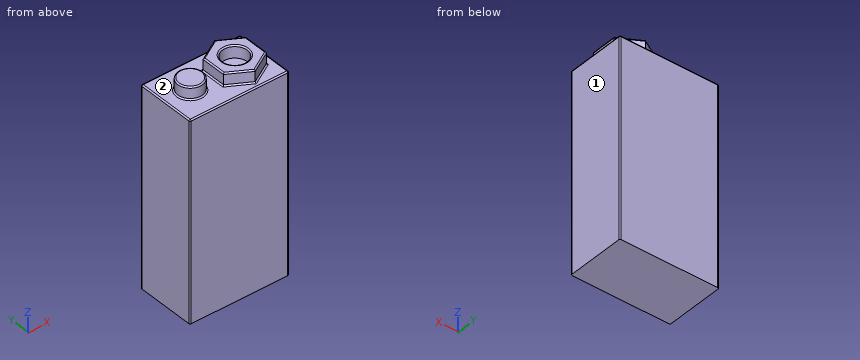
Autodesk Inventor part; units mm, degrees
ref_plane "YZ Plane" through (0, 0, 0) normal (1, 0, 0) x (0, 1, 0)
ref_plane "XZ Plane" through (0, 0, 0) normal (0, 1, 0) x (-1, 0, 0)
ref_plane "XY Plane" through (0, 0, 0) normal (0, 0, 1) x (1, 0, 0)
sketch "Sketch1" plane through (0, 0, 0) normal (0, 0, 1) x (1, 0, 0)
  line L0 (20, 12) -> (0, 12)
  line L1 (0, 12) -> (0, 0)
  line L2 (0, 0) -> (20, 0)
  line L3 (20, 0) -> (20, 12)
extrude "Extrusion1" add sketch "Sketch1" along normal blind 40
sketch "Sketch2" plane through (0, 0, 40) normal (0, 0, 1) x (1, 0, 0)
  circle A0 centre (5, 6) radius 2.5
  line L0 (14, 1) -> (9.6699, 3.5)
  line L1 (9.6699, 3.5) -> (9.6699, 8.5)
  line L2 (9.6699, 8.5) -> (14, 11)
  line L3 (14, 11) -> (18.3301, 8.5)
  line L4 (18.3301, 8.5) -> (18.3301, 3.5)
  line L5 (18.3301, 3.5) -> (14, 1)
  point P0 (0, 0)
  point P1 (14, 6)
extrude "Extrusion2" add sketch "Sketch2" along normal blind 2.5
sketch "Sketch3" plane through (0, 0, 42.5) normal (0, 0, 1) x (1, 0, 0)
  circle A0 centre (14, 6) radius 2.5
  point P0 (0, 0)
  dimension "d15" = 5
extrude "Extrusion3" cut sketch "Sketch3" against normal blind 2.5
fillet "Fillet1" radius 0.25 1 edges at (2.5, 6, 42.5)
fillet "Fillet2" radius 0.25 13 edges at (11.8349, 2.25, 42.5) (16.1651, 2.25, 42.5) (18.3301, 6, 42.5) (9.6699, 6, 42.5) (11.8349, 9.75, 42.5) (16.1651, 9.75, 42.5) (11.5, 6, 42.5) (16.1651, 2.25, 40) (11.8349, 2.25, 40) (18.3301, 6, 40) (16.1651, 9.75, 40) (9.6699, 6, 40) (11.8349, 9.75, 40)
fillet "Fillet3" radius 0.25 1 edges at (2.5, 6, 40)
fillet "Fillet4" radius 0.25 8 edges at (20, 0, 20) (20, 12, 20) (0, 12, 20) (0, 0, 20) (0, 6, 40) (10, 0, 40) (20, 6, 40) (10, 12, 40)
properties part number "SPARC BOT Battery"
Part model, mm, in its own coordinate system. Face numbers are marked on the shaded views. A direction names the side the tool comes from. Coordinates: 2 decimals unless noted, no trailing zeros. Write each loop counter-clockwise with the first axis right and the second up, starting at its lowest first coordinate (ties: lowest second). Pieces come first, ordered by that corner, then holes.
Item 1: Which spindle directions (+Z, -Z, +X, -X, +Y, -Y) get a long thin tool onto all of the face, cutting with end or side? Do the marked faces 1 and 2. Say none if no direction does.
Item 2: Slice it at B-B (x = 5). Write the cut outline in (y, z).
Item 3: Slice it at A-A (y = 6). Write the cut outline in (x, z), and give its area (3 significant figures).
Item 4: Slice it at C-C (x = 8.5). Write the cut outline in (y, z).
Item 5: Probe line 1 (Y direction, x = 14, z = 41.1); line 2 (Z direction, x = 3, y = 10.5); line 3 (X direction, y = 4.5, z = 40.5). List the from-to ranges inside material, lowest first.
Item 6: Pin check, flat tips, straight feed: pin 1 (1.6 mm diameter, centred on y = 6, z = 41.5, fed in from -X); pin 2 (1 mm diameter, centred on y = 5, z = 41, fed in from +X); pin 3 (1.5 mm diameter, centred on x = 14.5, y = 5, fed in from +Z). Stop position of each tip, or through.
Results found:
1. face 1: +Z, -Z, +X, +Y, -Y
1. face 2: +Z
2. outline: (0, 0) - (12, 0) - (12, 39.75) arc R0.25 ccw to (11.75, 40) - (8.75, 40) arc R0.25 cw to (8.5, 40.25) - (8.5, 42.25) arc R0.25 ccw to (8.25, 42.5) - (3.75, 42.5) arc R0.25 ccw to (3.5, 42.25) - (3.5, 40.25) arc R0.25 cw to (3.25, 40) - (0.25, 40) arc R0.25 ccw to (0, 39.75) - close
3. outline: (0, 0) - (20, 0) - (20, 39.75) arc R0.25 ccw to (19.75, 40) - (18.58, 40) arc R0.25 cw to (18.33, 40.25) - (18.33, 42.25) arc R0.25 ccw to (18.08, 42.5) - (16.75, 42.5) arc R0.25 ccw to (16.5, 42.25) - (16.5, 40) - (11.5, 40) - (11.5, 42.25) arc R0.25 ccw to (11.25, 42.5) - (9.92, 42.5) arc R0.25 ccw to (9.67, 42.25) - (9.67, 40.25) arc R0.25 cw to (9.42, 40) - (7.75, 40) arc R0.25 cw to (7.5, 40.25) - (7.5, 42.25) arc R0.25 ccw to (7.25, 42.5) - (2.75, 42.5) arc R0.25 ccw to (2.5, 42.25) - (2.5, 40.25) arc R0.25 cw to (2.25, 40) - (0.25, 40) arc R0.25 ccw to (0, 39.75) - close
3. area: 822 mm2
4. outline: (0, 0) - (12, 0) - (12, 39.75) arc R0.25 ccw to (11.75, 40) - (0.25, 40) arc R0.25 ccw to (0, 39.75) - close
5. line 1: y = 1 to 3.5, 8.5 to 11
5. line 2: z = 0 to 40
5. line 3: x = 3 to 7, 9.67 to 12, 16 to 18.33
6. pin 1: stops at x = 2.5
6. pin 2: stops at x = 18.33
6. pin 3: stops at z = 40
